Verification items for the finished model (mm, model axes). Face numbers are marked on the shaded views. A direction names the side the tool comes from. Give positions to 0.01 mm unless a question says otherwise; leave off trailing zeros. Order: outer loops, then holes, each group sorted by start corner. A loop starts at its lowest first (then second) coordinate and runs counter-clockwise, first axis right, second up. Notation, with made-up numbers: (-3.75, 30) -> (17.25, 30) arc R22 cw to (17.25, 64) -> close; hole circle Ø11 at (28.5, 36). An arc over 180 degrees is marked (long way). One line per question, with ' | ' between items. Start each with the question number.
Q1. Section check C-C on z = 4.2. Record the cut outline in (x, y) (3 decimals).
Q2. Section check D-D on y = 0. Record the cut outline in (x, z) (3 decimals), plus the area to 4 significant figures.
Q3. Section check B-B on x = 10. Record the cut outline in (y, z).
Q4. Access from +Z, -Z, +X, -X, +Y, -Y to the whole of each face (thin tool, end or side, straight path). Record for the marked faces 4 and 5.
Q5. Material ranges on probe 1 along Y at (x, z) = (0, 1.3) (3 decimals); probe 2 along X at (y, z) = (-10, 3); probe 3 along X at (y, z) = (-0.75, 4.85), recorded low to high. Write a range as [from, to].
Q6. Section check A-A on y = 10. Record the cut outline in (x, z), plus the area to 4 significant figures.
Q7. Go/stop test with flat-tipped pins: pin 1 (3 mm diameter, centred on x = -1, y = -11, fed in from +Z); pin 2 (2 mm diameter, centred on x = 2.5, y = 0.5, fed in from +Z). Record where each tip stops, or that it passes through.
Q8. Mould release check, pull along Y, two halves, no side actions. Record for the marked faces 1, 2 and 3: released by +Y, released by -Y, zero draft, split by the parting line, or undercut.
from build123d import *

# Parameters (mm, degrees)
SKETCH1_W           = 30
SKETCH1_H           = 30
SKETCH1_R           = 4.725
BOSS_EXTRUDE1_DEPTH = 5
FILLET1_R           = 2
SKETCH2_R           = 1.75
CUT_EXTRUDE1_DEPTH  = 22.794494718
CIRPATTERN1_COUNT   = 4
SKETCH3_R           = 3.25
CUT_EXTRUDE2_DEPTH  = 2.5
CIRPATTERN2_COUNT   = 4
SKETCH4_W           = 1
SKETCH4_H           = 5
CUT_EXTRUDE3_DEPTH  = 2.5


with BuildPart() as part:
    # Sketch1 → Boss-Extrude1 (new body)
    with BuildSketch(Plane.XY):
        Rectangle(SKETCH1_W, SKETCH1_H)
        Circle(SKETCH1_R, mode=Mode.SUBTRACT)
    extrude(amount=BOSS_EXTRUDE1_DEPTH)

    # Fillet1
    fillet1_edges = [part.edges().sort_by_distance(p)[0] for p in [
        (-15, 15, 2.5),
        (15, 15, 2.5),
        (15, -15, 2.5),
        (-15, -15, 2.5),
    ]]
    fillet(fillet1_edges, radius=FILLET1_R)

    # Sketch2 → Cut-Extrude1 (cut, symmetric)
    with BuildSketch(Plane.XY):
        with Locations((0, 10)):
            Circle(SKETCH2_R)
    cut_extrude1 = extrude(amount=CUT_EXTRUDE1_DEPTH, both=True, mode=Mode.SUBTRACT)

    # CirPattern1: Cut-Extrude1 ×4 about axis
    cirpattern1_axis = Axis((0, 0, 0), (0, 0, 1))
    for i in range(1, CIRPATTERN1_COUNT):
        add(cut_extrude1.rotate(cirpattern1_axis, i * 360 / CIRPATTERN1_COUNT), mode=Mode.SUBTRACT)

    # Sketch3 → Cut-Extrude2 (cut)
    with BuildSketch(Plane.XY.offset(5)):
        with Locations((0, 10)):
            Circle(SKETCH3_R)
    cut_extrude2 = extrude(amount=-CUT_EXTRUDE2_DEPTH, mode=Mode.SUBTRACT)

    # CirPattern2: Cut-Extrude2 ×4 about axis
    cirpattern2_axis = Axis((0, 0, 0), (0, 0, 1))
    for i in range(1, CIRPATTERN2_COUNT):
        add(cut_extrude2.rotate(cirpattern2_axis, i * 360 / CIRPATTERN2_COUNT), mode=Mode.SUBTRACT)

    # Sketch4 → Cut-Extrude3 (cut)
    with BuildSketch(Plane.XY.offset(5)):
        with Locations((-11, 9)):
            Rectangle(SKETCH4_W, SKETCH4_H)
    extrude(amount=-CUT_EXTRUDE3_DEPTH, mode=Mode.SUBTRACT)


solid = part.part
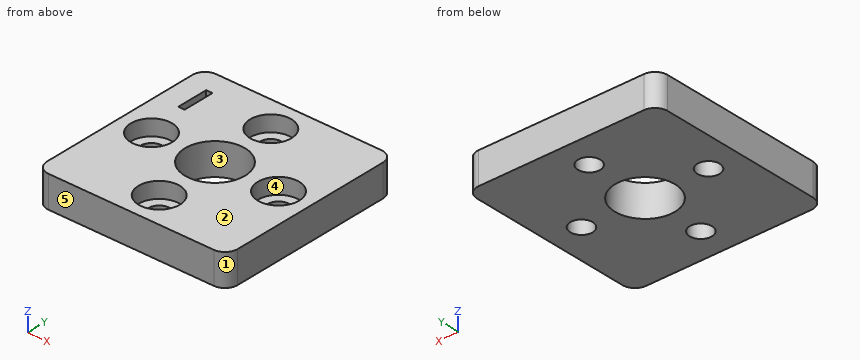
Filled in:
1) outline: (-15, -13) arc R2 ccw to (-13, -15) -> (13, -15) arc R2 ccw to (15, -13) -> (15, 13) arc R2 ccw to (13, 15) -> (-13, 15) arc R2 ccw to (-15, 13) -> close; hole circle Ø6.5 at (-10, 0); hole (-11.5, 6.5) -> (-10.5, 6.5) -> (-10.5, 11.5) -> (-11.5, 11.5) -> close; hole circle Ø9.45 at (0, 0); hole circle Ø6.5 at (0, -10); hole circle Ø6.5 at (0, 10); hole circle Ø6.5 at (10, 0)
2) outline: (-15, 0) -> (-11.75, 0) -> (-11.75, 2.5) -> (-13.25, 2.5) -> (-13.25, 5) -> (-15, 5) -> close; (-8.25, 0) -> (-4.725, 0) -> (-4.725, 5) -> (-6.75, 5) -> (-6.75, 2.5) -> (-8.25, 2.5) -> close; (4.725, 0) -> (8.25, 0) -> (8.25, 2.5) -> (6.75, 2.5) -> (6.75, 5) -> (4.725, 5) -> close; (11.75, 0) -> (15, 0) -> (15, 5) -> (13.25, 5) -> (13.25, 2.5) -> (11.75, 2.5) -> close | area: 52.75 mm²
3) outline: (-15, 0) -> (-1.75, 0) -> (-1.75, 2.5) -> (-3.25, 2.5) -> (-3.25, 5) -> (-15, 5) -> close; (1.75, 0) -> (15, 0) -> (15, 5) -> (3.25, 5) -> (3.25, 2.5) -> (1.75, 2.5) -> close
4) face 4: +Z | face 5: +Z, -Z, +X, -X, -Y
5) probe 1: [-15, -11.75], [-8.25, -4.725], [4.725, 8.25], [11.75, 15] | probe 2: [-15, -3.25], [3.25, 15] | probe 3: [-15, -13.16], [-6.84, -4.67], [4.67, 6.84], [13.16, 15]
6) outline: (-15, 0) -> (-1.75, 0) -> (-1.75, 2.5) -> (-3.25, 2.5) -> (-3.25, 5) -> (-10.5, 5) -> (-10.5, 2.5) -> (-11.5, 2.5) -> (-11.5, 5) -> (-15, 5) -> close; (1.75, 0) -> (15, 0) -> (15, 5) -> (3.25, 5) -> (3.25, 2.5) -> (1.75, 2.5) -> close | area: 122.5 mm²
7) pin 1: z = 2.5 | pin 2: through
8) face 1: released by -Y | face 2: zero draft | face 3: undercut
